Work out the finished part from the listing and answer in its coordinate system (mm). Face numbers are marked on the shaded views. A direction names the side the tool comes from. Coordinates: 2 decimals unless noted, no trailing zeros. Write each loop counter-clockwise with the first axis right and the second up, starting at its lowest first coordinate (ties: lowest second). Pieces come first, ordered by that corner, then holes. Notation, with made-up numbers: (71.25, -27.75) - (105.25, -27.75) arc R22 cw to (105.25, -18.75) - close; hole circle Ø9 at (41.25, 19.5). An arc over 180 degrees is marked (long way). One line per item, written item: value.
```python
from build123d import *

# Parameters (mm, degrees)
SKETCH_1_W          = 94
SKETCH_1_H          = 26
SKETCH_1_R          = 1
EXTRUDE_1_DEPTH     = 0.8
SKETCH_3_W          = 15.4
SKETCH_3_H          = 15.1
EXTRUDE_4_DEPTH     = 1.9
SKETCH_3_3_W        = 6.7
SKETCH_3_3_H        = 6.2
EXTRUDE_5_DEPTH     = 1
SKETCH_3_4_W        = 8.4
SKETCH_3_4_H        = 5.9
EXTRUDE_6_DEPTH     = 1.5
SKETCH_3_5_W        = 7.6
SKETCH_3_5_H        = 5.9
EXTRUDE_7_DEPTH     = 2.5
SKETCH_3_6_W        = 4.5
SKETCH_3_6_H        = 8.7
CUT_EXTRUDE_1_DEPTH = 49.828782496


with BuildPart() as part:
    # Sketch 1 → Extrude 1 (new body)
    with BuildSketch(Plane(origin=(0, 0, 0), x_dir=(1, 0, 0), z_dir=(0, 1, 0))):
        Rectangle(SKETCH_1_W, SKETCH_1_H)
        with Locations(Location((-44, 10, 0), (0, 0, 270))):
            Circle(SKETCH_1_R, mode=Mode.SUBTRACT)
        with Locations(Location((-44, -10, 0), (0, 0, 270))):
            Circle(SKETCH_1_R, mode=Mode.SUBTRACT)
        with Locations(Location((44, 10, 0), (0, 0, 270))):
            Circle(SKETCH_1_R, mode=Mode.SUBTRACT)
        with Locations(Location((44, -10, 0), (0, 0, 270))):
            Circle(SKETCH_1_R, mode=Mode.SUBTRACT)
    extrude(amount=EXTRUDE_1_DEPTH)

    # Sketch 3 → Extrude 4 (add)
    with BuildSketch(Plane.XZ):
        with Locations((32.9, 5.45)):
            Rectangle(SKETCH_3_W, SKETCH_3_H)
    extrude(amount=EXTRUDE_4_DEPTH)

    # Sketch 3_3 → Extrude 5 (add)
    with BuildSketch(Plane.XZ):
        with Locations((-27.35, 0)):
            Rectangle(SKETCH_3_3_W, SKETCH_3_3_H)
        with Locations((-16.075, 0)):
            Rectangle(SKETCH_3_3_W, SKETCH_3_3_H)
        with Locations((-4.8, 0)):
            Rectangle(SKETCH_3_3_W, SKETCH_3_3_H)
        with Locations((6.475, 0)):
            Rectangle(SKETCH_3_3_W, SKETCH_3_3_H)
        with Locations((17.75, 0)):
            Rectangle(SKETCH_3_3_W, SKETCH_3_3_H)
    extrude(amount=EXTRUDE_5_DEPTH)

    # Sketch 3_4 → Extrude 6 (add)
    with BuildSketch(Plane.XZ):
        with Locations((-27.5, 10.05)):
            Rectangle(SKETCH_3_4_W, SKETCH_3_4_H)
    extrude(amount=EXTRUDE_6_DEPTH)

    # Sketch 3_5 → Extrude 7 (add)
    with BuildSketch(Plane.XZ):
        with Locations((-37.2, 10.05)):
            Rectangle(SKETCH_3_5_W, SKETCH_3_5_H)
    extrude(amount=EXTRUDE_7_DEPTH)

    # Sketch 3_6 → Cut-Extrude 1 (cut, through all)
    with BuildSketch(Plane.XZ):
        with Locations((-44.75, 2.65)):
            Rectangle(SKETCH_3_6_W, SKETCH_3_6_H)
    extrude(amount=-CUT_EXTRUDE_1_DEPTH, mode=Mode.SUBTRACT)


solid = part.part
```
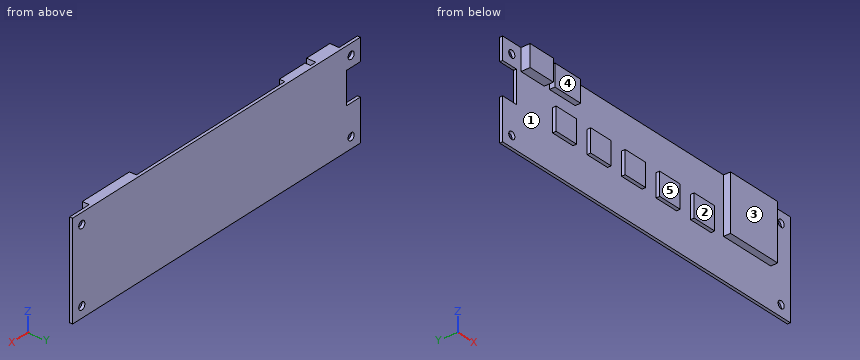
Item 1: Determine the mould class of the marked faces 1 and 2 for opening direction X: +X half, -X half, draft (parallel to the pull), parting line (faces both ways), or undercut.
Evaluation:
face 1: undercut
face 2: draft
Item 2: Section C-C, the plane x = -44 is taken. Determine the outline of the cut face in (y, z), then the cut area to 3 significant figures.
Evaluation:
outline: (0, -13) - (0.8, -13) - (0.8, -11) - (0, -11) - close; (0, -9) - (0.8, -9) - (0.8, -1.7) - (0, -1.7) - close; (0, 7) - (0.8, 7) - (0.8, 9) - (0, 9) - close; (0, 11) - (0.8, 11) - (0.8, 13) - (0, 13) - close
area: 10.6 mm2
Item 3: Section A-A, the plane x = 44 is taken. Determine the outline of the cut face in (y, z).
Evaluation:
outline: (0, -13) - (0.8, -13) - (0.8, -11) - (0, -11) - close; (0, -9) - (0.8, -9) - (0.8, 9) - (0, 9) - close; (0, 11) - (0.8, 11) - (0.8, 13) - (0, 13) - close
Item 4: Section B-B, the plane z = -10 is taken. Determine the outline of the cut face in (x, y), then the cut area to 3 significant figures.
Evaluation:
outline: (-47, 0) - (-45, 0) - (-45, 0.8) - (-47, 0.8) - close; (-43, 0) - (43, 0) - (43, 0.8) - (-43, 0.8) - close; (45, 0) - (47, 0) - (47, 0.8) - (45, 0.8) - close
area: 72.0 mm2
Item 5: Section D-D, the plane z = 10 is taken. Determine the outline of the cut face in (x, y), then the cut area to 3 significant figures.
Evaluation:
outline: (-47, 0) - (-45, 0) - (-45, 0.8) - (-47, 0.8) - close; (-43, 0) - (-41, 0) - (-41, -2.5) - (-33.4, -2.5) - (-33.4, 0) - (-31.7, 0) - (-31.7, -1.5) - (-23.3, -1.5) - (-23.3, 0) - (25.2, 0) - (25.2, -1.9) - (40.6, -1.9) - (40.6, 0) - (43, 0) - (43, 0.8) - (-43, 0.8) - close; (45, 0) - (47, 0) - (47, 0.8) - (45, 0.8) - close
area: 133 mm2
Item 6: Given pin 1 (0.8 mm diameter, centred on x = -25.5, y = -1, fed in from -Z); pin 2 (0.8 mm diameter, centred on y = -0.5, z = -1.5, fed in from +X); pin 3 (5 mm diameter, centred on x = 8.5, z = 0.5, fed in from -Y), each flat-ended and moving along its own axis, determine where each tip first touches the part or whether it passes through.
Evaluation:
pin 1: stops at z = -3.1
pin 2: stops at x = 40.6
pin 3: stops at y = -1
Item 7: Which of the six approach directions +Z, -Z, +X, -X, +Y, -Y give full straight-line access (tool end or side, diameter ignored) to the marked faces 3, 4 and 5?
Evaluation:
face 3: +Z, -Z, +X, -Y
face 4: +Z, -Z, -Y
face 5: +Z, -Z, -X, -Y
Item 8: Consider probe 1 along X at (y, z) = (-0.85, 2) (3 decimals); probe 2 along X at (y, z) = (0.5, 10); probe 3 along X at (y, z) = (-1.75, 11.5). Determine where each line is inside the solid, lowest interval first.
Evaluation:
probe 1: x = -30.7 to -24, -19.425 to -12.725, -8.15 to -1.45, 3.125 to 9.825, 14.4 to 21.1, 25.2 to 40.6
probe 2: x = -47 to -45, -43 to 43, 45 to 47
probe 3: x = -41 to -33.4, 25.2 to 40.6
